```python
from build123d import *

# Parameters (mm, degrees)
SKETCH1_W                                         = 76.2
SKETCH1_H                                         = 12.7
BOSS_EXTRUDE2_DEPTH                               = 4.7625
CSK_FOR_4_FLAT_HEAD_SOCKET_CAP_SCREW1_D           = 3.2639
CSK_FOR_4_FLAT_HEAD_SOCKET_CAP_SCREW1_CSINK_D     = 6.477
CSK_FOR_4_FLAT_HEAD_SOCKET_CAP_SCREW1_CSINK_ANGLE = 82
CUT_EXTRUDE1_DEPTH                                = 5.7625
CHAMFER1_SIZE                                     = 0.508


with BuildPart() as part:
    # Sketch1 → Boss-Extrude2 (new body)
    with BuildSketch(Plane(origin=(0, 0, 0), x_dir=(1, 0, 0), z_dir=(0, 1, 0))):
        with Locations((-31.75, 0)):
            Rectangle(SKETCH1_W, SKETCH1_H)
    extrude(amount=BOSS_EXTRUDE2_DEPTH)

    # CSK for #4 Flat Head Socket Cap Screw1 (through all)
    with Locations(Plane(origin=(0, 4.7625, 0), x_dir=(1, 0, 0), z_dir=(0, 1, 0))):
        with Locations((-63.5, 0)):
            CounterSinkHole(CSK_FOR_4_FLAT_HEAD_SOCKET_CAP_SCREW1_D / 2, CSK_FOR_4_FLAT_HEAD_SOCKET_CAP_SCREW1_CSINK_D / 2, counter_sink_angle=CSK_FOR_4_FLAT_HEAD_SOCKET_CAP_SCREW1_CSINK_ANGLE)

    # Sketch2 → Cut-Extrude1 (cut, through all)
    with BuildSketch(Plane(origin=(0, 4.7625, 0), x_dir=(1, 0, 0), z_dir=(0, 1, 0))):
        with BuildLine():
            ThreePointArc((3.1623, 0), (2.236083774, 2.236083774), (0, 3.1623))
            Line((0, 3.1623), (0, -3.1623))
            ThreePointArc((0, -3.1623), (2.236083774, -2.236083774), (3.1623, 0))
        make_face()
        with BuildLine():
            Line((0, -3.1623), (0, 3.1623))
            ThreePointArc((0, 3.1623), (-3.1623, 0), (0, -3.1623))
        make_face()
    extrude(amount=-CUT_EXTRUDE1_DEPTH, mode=Mode.SUBTRACT)

    # Chamfer1
    chamfer1_edges = [part.edges().sort_by_distance(p)[0] for p in [
        (-69.85, 2.38125, 6.35),
        (-69.85, 2.38125, -6.35),
        (6.35, 2.38125, -6.35),
        (6.35, 2.38125, 6.35),
        (6.35, 4.7625, 0),
        (-69.85, 4.7625, 0),
        (-69.85, 0, 0),
        (6.35, 0, 0),
    ]]
    chamfer(chamfer1_edges, length=CHAMFER1_SIZE)


solid = part.part
```
Read the model definition and answer for the solid it produces. Units are mm, in the model's axes. Coordinates: 2 decimals unless noted, no trailing zeros. Loops run counter-clockwise (first coordinate to the right, second up) from the corner with the lowest first, then second, coordinate; pieces in that order, holes last.
(1) The part is cut by section A-A (x = -63.5). Determine the outline of the cut face in (y, z).
Solution:
outline: (0, -6.35) - (4.76, -6.35) - (4.76, -3.24) - (2.91, -1.63) - (0, -1.63) - close; (0, 1.63) - (2.91, 1.63) - (4.76, 3.24) - (4.76, 6.35) - (0, 6.35) - close
(2) Consider line 1 along Z through (x, y) = (-63.5, 1.3); line 2 along Y through (x, z) = (-64.5, 1.75). Determine where each line is inside the solid, lowest interval first.
Solution:
line 1: z = -6.35 to -1.63, 1.63 to 6.35
line 2: y = 0 to 3.36
(3) The mould has two halves that part along X. Classify faces 1 (the face through (-32, 4.762, 0)), 2 (the face through (-61.87, 1.44, -0.07)), 3 (the face through (6.35, 2, 0)), 4 (the face through (-69.85, 2, 0)): released by +X, released by -X, zero draft, split by the parting line, or undercut.
Solution:
face 1: zero draft
face 2: undercut
face 3: released by +X
face 4: released by -X
(4) The part is cut by section C-C (z = 1). Count the separate pieces of the cut face and the enclosed holes in it, and give its area (3 significant figures).
Solution:
separate pieces: 3
enclosed holes: 0
area: 318 mm2
(5) The part is cut by section B-B (y = 3.6). Determine the outline of the cut face in (x, z).
Solution:
outline: (-69.85, -5.84) - (-69.34, -6.35) - (5.84, -6.35) - (6.35, -5.84) - (6.35, 5.84) - (5.84, 6.35) - (-69.34, 6.35) - (-69.85, 5.84) - close; hole circle Ø4.46 at (-63.5, 0); hole circle Ø6.32 at (0, 0)
